```python
from build123d import *

# Parameters (mm, degrees)
SKETCH1_R                                            = 1.5875
BOSS_EXTRUDE1_DEPTH                                  = 3
SKETCH2_R                                            = 2.1
CUT_EXTRUDE1_DEPTH                                   = 94.949837679
BOSS_EXTRUDE2_START                                  = 4
SKETCH3_R                                            = 4
SKETCH3_R_2                                          = 2.1
BOSS_EXTRUDE2_DEPTH                                  = 4
CSK_FOR_M3_HEX_SOCKET_COUNTERSUNK_CAP_SC_D           = 3.6
CSK_FOR_M3_HEX_SOCKET_COUNTERSUNK_CAP_SC_DEPTH       = 14.44
CSK_FOR_M3_HEX_SOCKET_COUNTERSUNK_CAP_SC_CSINK_D     = 6.72
CSK_FOR_M3_HEX_SOCKET_COUNTERSUNK_CAP_SC_CSINK_ANGLE = 90
CSK_FOR_M3_HEX_SOCKET_COUNTERSUNK_CAP_SC_TIP         = 1.081549114


with BuildPart() as part:
    # Sketch1 → Boss-Extrude1 (new body)
    with BuildSketch(Plane(origin=(0, 0, 0), x_dir=(1, 0, 0), z_dir=(0, 1, 0))):
        Polygon((5, -5), (5, 71.04), (-0.468932188, 71.04), (-3.008932188, 73.58), (-39.917067812, 73.58), (-42.457067812, 71.04), (-58.34, 71.04), (-58.34, -5), align=None)
        with Locations(Location((-50.8, 15.24, 0), (0, 0, 270))):
            Circle(SKETCH1_R, mode=Mode.SUBTRACT)
        with Locations(Location((-2.54, 13.97, 0), (0, 0, 270))):
            Circle(SKETCH1_R, mode=Mode.SUBTRACT)
        with Locations(Location((-7.62, 66.04, 0), (0, 0, 270))):
            Circle(SKETCH1_R, mode=Mode.SUBTRACT)
        with Locations(Location((-35.56, 66.04, 0), (0, 0, 270))):
            Circle(SKETCH1_R, mode=Mode.SUBTRACT)
    extrude(amount=BOSS_EXTRUDE1_DEPTH)

    # Sketch2 → Cut-Extrude1 (cut, through all)
    with BuildSketch(Plane(origin=(0, 3, 0), x_dir=(1, 0, 0), z_dir=(0, 1, 0))):
        with Locations(Location((-50.8, 15.24, 0), (0, 0, 270))):
            Circle(SKETCH2_R)
        with Locations(Location((-35.56, 66.04, 0), (0, 0, 270))):
            Circle(SKETCH2_R)
        with Locations(Location((-7.62, 66.04, 0), (0, 0, 270))):
            Circle(SKETCH2_R)
        with Locations(Location((-2.54, 13.97, 0), (0, 0, 270))):
            Circle(SKETCH2_R)
    extrude(amount=-CUT_EXTRUDE1_DEPTH, mode=Mode.SUBTRACT)

    # Sketch3 → Boss-Extrude2 (add)
    # profile 1 of 4: a face of its own
    with BuildSketch(Plane(origin=(0, 3, 0), x_dir=(1, 0, 0), z_dir=(0, 1, 0)).offset(BOSS_EXTRUDE2_START)):
        with Locations(Location((-50.8, 15.24, 0), (0, 0, 270))):
            Circle(SKETCH3_R)
        with Locations(Location((-50.8, 15.24, 0), (0, 0, 270))):
            Circle(SKETCH3_R_2, mode=Mode.SUBTRACT)
    # profile 2 of 4: a face of its own
    with BuildSketch(Plane(origin=(0, 3, 0), x_dir=(1, 0, 0), z_dir=(0, 1, 0)).offset(BOSS_EXTRUDE2_START)):
        with Locations(Location((-35.56, 66.04, 0), (0, 0, 270))):
            Circle(SKETCH3_R)
        with Locations(Location((-35.56, 66.04, 0), (0, 0, 270))):
            Circle(SKETCH3_R_2, mode=Mode.SUBTRACT)
    # profile 3 of 4: a face of its own
    with BuildSketch(Plane(origin=(0, 3, 0), x_dir=(1, 0, 0), z_dir=(0, 1, 0)).offset(BOSS_EXTRUDE2_START)):
        with Locations(Location((-7.62, 66.04, 0), (0, 0, 270))):
            Circle(SKETCH3_R)
        with Locations(Location((-7.62, 66.04, 0), (0, 0, 270))):
            Circle(SKETCH3_R_2, mode=Mode.SUBTRACT)
    # profile 4 of 4: a face of its own
    with BuildSketch(Plane(origin=(0, 3, 0), x_dir=(1, 0, 0), z_dir=(0, 1, 0)).offset(BOSS_EXTRUDE2_START)):
        with Locations(Location((-2.54, 13.97, 0), (0, 0, 270))):
            Circle(SKETCH3_R)
        with Locations(Location((-2.54, 13.97, 0), (0, 0, 270))):
            Circle(SKETCH3_R_2, mode=Mode.SUBTRACT)
    extrude(amount=-BOSS_EXTRUDE2_DEPTH)

    # CSK for M3 Hex Socket Countersunk Cap Screw1
    with Locations(Plane(origin=(0, 3, 0), x_dir=(1, 0, 0), z_dir=(0, 1, 0))):
        with Locations((-34.797780841, 44.973541217), (-19.797780841, 44.973541217)):
            CounterSinkHole(CSK_FOR_M3_HEX_SOCKET_COUNTERSUNK_CAP_SC_D / 2, CSK_FOR_M3_HEX_SOCKET_COUNTERSUNK_CAP_SC_CSINK_D / 2, depth=CSK_FOR_M3_HEX_SOCKET_COUNTERSUNK_CAP_SC_DEPTH, counter_sink_angle=CSK_FOR_M3_HEX_SOCKET_COUNTERSUNK_CAP_SC_CSINK_ANGLE)
            with Locations((0, 0, -(CSK_FOR_M3_HEX_SOCKET_COUNTERSUNK_CAP_SC_DEPTH + CSK_FOR_M3_HEX_SOCKET_COUNTERSUNK_CAP_SC_TIP / 2))):  # 118° drill point
                Cone(0, CSK_FOR_M3_HEX_SOCKET_COUNTERSUNK_CAP_SC_D / 2, CSK_FOR_M3_HEX_SOCKET_COUNTERSUNK_CAP_SC_TIP, mode=Mode.SUBTRACT)


solid = part.part
```
Work out the finished part from the listing and answer in its coordinate system (mm). A direction names the side the tool comes from. Give positions to 0.01 mm unless a question says otherwise; leave off trailing zeros. Loops run counter-clockwise (first coordinate to the right, second up) from the corner with the lowest first, then second, coordinate; pieces in that order, holes last. Notation, with made-up numbers: M 44.5,-5 L 77.5,-5 A14 ccw 77.5,1 Z; hole C 89.5,41.25 d2. An arc over 180 degrees is marked long. One line per item, written item: value. Start each with the question number.
1. Find section B-B (y = 4.5). Give the vertices of the cut face in (x, z).
2. Find the intervals of material crossed by probe 1 along X at (y, z) = (3.5, -66.04); probe 2 along X at (y, z) = (2, -13.97); probe 3 along Y at (x, z) = (-11, -44.5), in increasing order.
3. Determine the mould class of faces 1 (the face through (-27, 0, -35)), 2 (the face through (-9.152, 5.028, -62.345)), 3 (the face through (2, 1, -71.04)), 4 (the face through (-54.349, 5.028, -13.394)) for opening direction Z: released by +Z, released by -Z, zero draft, split by the parting line, or undercut.
4. Which of the six approach directions +Z, -Z, +X, -X, +Y, -Y give full straight-line access (tool end or side, diameter ignored) to faces 5 (the face through (-9, 7, -64)), 6 (the face through (-1.339, 5.028, -10.155))?
5. Each of these flat-tipped pins is pushed along its axis until it touches: P1, Ø1.5, axis at x = -34, z = -12, coming from the +Y side; P2, Ø1, axis at x = -52, y = 6, coming from the -Z side; P3, Ø4.5, axis at x = -34.8, z = -44.97, coming from the +Y side; P4, Ø5, axis at x = -50.8, z = -15.24, coming from the +Y side. Where does it stop, or does it pass through?
6. Find section D-D (x = -7.62). Give the vertices of the cut face in (y, z).
7. Find section C-C (z = -15.24). Give the vertices of the cut face in (x, y), and give its area (3 significant figures).
8. Find section A-A (x = -50.8). Give the vertices of the cut face in (y, z), and give its area (3 significant figures).
Reported:
1. outline: C -50.8,-15.24 d8; C -35.56,-66.04 d8; C -7.62,-66.04 d8; C -2.54,-13.97 d8; hole C -50.8,-15.24 d4.2; hole C -35.56,-66.04 d4.2; hole C -7.62,-66.04 d4.2; hole C -2.54,-13.97 d4.2
2. probe 1: x = -39.56 to -37.66, -33.46 to -31.56, -11.62 to -9.72, -5.52 to -3.62
2. probe 2: x = -58.34 to -52.47, -49.13 to -4.64, -0.44 to 5
2. probe 3: y = 0 to 3
3. face 1: zero draft
3. face 2: undercut
3. face 3: released by -Z
3. face 4: split by the parting line
4. face 5: +Z, -Z, +X, -X, +Y
4. face 6: +Y
5. P1: stops at y = 3
5. P2: stops at z = -19.18
5. P3: stops at y = 1.89
5. P4: stops at y = 7
6. outline: M 0,-73.58 L 3,-73.58 L 3,-70.04 L 7,-70.04 L 7,-68.14 L 0,-68.14 Z; M 0,-63.94 L 7,-63.94 L 7,-62.04 L 3,-62.04 L 3,5 L 0,5 Z
7. outline: M -58.34,0 L -52.9,0 L -52.9,7 L -54.8,7 L -54.8,3 L -58.34,3 Z; M -48.7,0 L -4.21,0 L -4.21,7 L -6.33,7 L -6.33,3 L -46.8,3 L -46.8,7 L -48.7,7 Z; M -0.87,0 L 5,0 L 5,3 L 1.25,3 L 1.25,7 L -0.87,7 Z
7. area: 200 mm²
8. outline: M 0,-71.04 L 3,-71.04 L 3,-19.24 L 7,-19.24 L 7,-17.34 L 0,-17.34 Z; M 0,-13.14 L 7,-13.14 L 7,-11.24 L 3,-11.24 L 3,5 L 0,5 Z
8. area: 231 mm²
